from build123d import *

# Parameters (mm, degrees)
SKETCH1_W           = 15
SKETCH1_H           = 15
SKETCH1_R           = 3
BOSS_EXTRUDE1_DEPTH = 24
SKETCH1_3_W         = 45
SKETCH1_3_H         = 25
SKETCH1_3_R         = 3
BOSS_EXTRUDE2_DEPTH = 10
CUT_EXTRUDE1_DEPTH  = 57.797887285
FILLET2_R           = 10


with BuildPart() as part:
    # Sketch1 → Boss-Extrude1 (new body)
    with BuildSketch(Plane.XY):
        with Locations((7.5, 17.5)):
            Rectangle(SKETCH1_W, SKETCH1_H)
        with Locations((10, 15)):
            Circle(SKETCH1_R, mode=Mode.SUBTRACT)
    extrude(amount=-BOSS_EXTRUDE1_DEPTH)

    # Sketch1<3> → Boss-Extrude2 (add)
    with BuildSketch(Plane.XY):
        with Locations((22.5, 12.5)):
            Rectangle(SKETCH1_3_W, SKETCH1_3_H)
        with Locations((10, 15)):
            Circle(SKETCH1_3_R, mode=Mode.SUBTRACT)
        with Locations((40, 10)):
            Circle(SKETCH1_3_R, mode=Mode.SUBTRACT)
    extrude(amount=-BOSS_EXTRUDE2_DEPTH)

    # Sketch2 → Cut-Extrude1 (cut, through all)
    with BuildSketch(Plane(origin=(45, 0, 0), x_dir=(0, 0, -1), z_dir=(1, 0, 0))):
        Polygon((0, 0), (3.513520868, 25), (0, 25), align=None)
    extrude(amount=-CUT_EXTRUDE1_DEPTH, mode=Mode.SUBTRACT)

    # Fillet2
    fillet2_edges = [part.edges().sort_by_distance(p)[0] for p in [
        (7.5, 10, -10),
        (15, 17.5, -10),
    ]]
    fillet(fillet2_edges, radius=FILLET2_R - 0.0001)  # a hair under: the kernel refuses the full size


solid = part.part
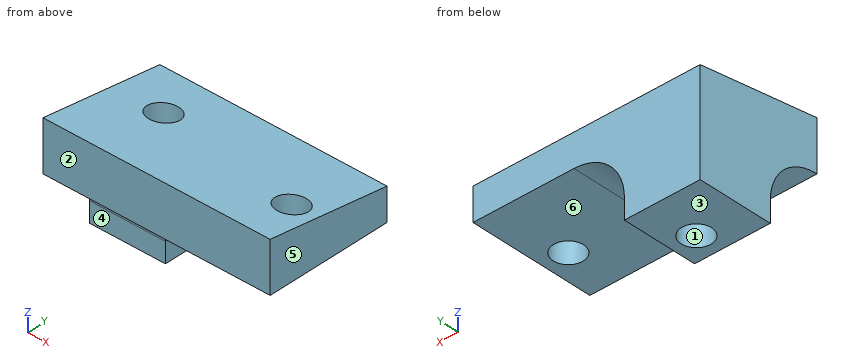
Can you work these out from the model? Positions are in its coordinate system, mm. Face numbers are marked on the shaded views. A direction names the side the tool comes from. Coordinates: 2 decimals unless noted, no trailing zeros. Write each loop counter-clockwise with the first axis right and the second up, starting at its lowest first coordinate (ties: lowest second). Pieces come first, ordered by that corner, then holes. Notation, with made-up numbers: (-6, 9) -> (11, 9) arc R18 cw to (11, 24) -> close; hole circle Ø2 at (15, -20.5). An arc over 180 degrees is marked (long way). Answer as CSV lines item,"result".
1) If I drill on line 1 (X direction, y = 10, z = -7.25); line 2 (Y direction, x = 40, z = -7); line 3 (X direction, y = 15, z = -8.5), over which ranges is the centre line in solid material (lowest first)? Write a range as from..to.
Check result:
line 1,"0..37, 43..45"
line 2,"0..7, 13..25"
line 3,"0..7, 13..45"
2) On a 3-axis mill with a long thin cutter (end or side, diameter ignored), from which of +Z, -Z, +X, -X, +Y, -Y can I reach the whole of each face in a straight line? I mean the marked faces 4, 5 and 6. Say none if no direction works.
Check result:
face 4,"-Z, +X, -X, -Y"
face 5,"+Z, -Z, +X, +Y, -Y"
face 6,"-Z, +X, +Y, -Y"
3) If we section it at B-B on y = 16.25: Please give me the cut outline in (x, z), then the cut area to 3 significant figures.
Check result:
outline,"(0, -24) -> (7.27, -24) -> (7.27, -2.28) -> (0, -2.28) -> close; (12.73, -24) -> (15, -24) -> (15, -20) arc R10 cw to (25, -10) -> (45, -10) -> (45, -2.28) -> (12.73, -2.28) -> close"
area,"460 mm²"
4) If we mould it in two halves opening along Y, with no side actions, what happens to the marked faces 1, 2 and 3? For each: +Y half, -Y half, draft (parallel to the pull), parting line (faces both ways), or undercut.
Check result:
face 1,"undercut"
face 2,"-Y half"
face 3,"draft"
5) If we section it at C-C on z = -11.5: Please give me the cut outline in (x, y).
Check result:
outline,"(0, 5.27) -> (19.73, 5.27) -> (19.73, 25) -> (0, 25) -> close; hole circle Ø6 at (10, 15)"
6) Will these pins go through, and if not, where does the flat tip stop? P1, Ø12, axis at y = 18.5, z = -20.5, coming from the +X side; P2, Ø3, axis at y = 20.5, z = -21, coming from the +X side; P3, Ø9.5, axis at x = 10, y = 15, coming from the +Z side; P4, Ø12, axis at x = 24, z = -17, coming from the -Y side.
Check result:
P1,"x = 16.65"
P2,"x = 15.01"
P3,"z = -1.44"
P4,"through"
7) If we section it at D-D on x = 30.5: Please give me the cut outline in (y, z), then the cut area to 3 significant figures.
Check result:
outline,"(0, -10) -> (25, -10) -> (25, -3.51) -> (0, 0) -> close"
area,"206 mm²"
